from build123d import *

# Parameters (mm, degrees)
F0_R     = 1
F1_DEPTH = 1
F2_R     = 3
F3_W     = 1.5266574919
F3_H     = 4.5481626876
F4_DEPTH = 0.5
F5_R     = 0.5


with BuildPart() as f1:
    # F0 (on Top) → F1 (new body)
    with BuildSketch(Plane.XY):
        with BuildLine():
            ThreePointArc((-35.1311429143, -3.4115522057), (-32.1311429143, -6.4115522057), (-29.1311429143, -3.4115522057))
            Line((-29.1311429143, -3.4115522057), (-35.1311429143, -3.4115522057))
        make_face()
        with BuildLine():
            Line((-35.1311429143, -3.4115522057), (-29.1311429143, -3.4115522057))
            ThreePointArc((-29.1311429143, -3.4115522057), (-32.1311429143, -0.4115522057), (-35.1311429143, -3.4115522057))
        make_face()
        with Locations((-32.1311429143, -2.1592592821)):
            Circle(F0_R, mode=Mode.SUBTRACT)
        with BuildLine():
            Line((-25.6311429143, -3.4115522057), (-29.1311429143, -3.4115522057))
            ThreePointArc((-29.1311429143, -3.4115522057), (-32.1311429143, -6.4115522057), (-35.1311429143, -3.4115522057))
            Line((-35.1311429143, -3.4115522057), (-38.6311429143, -3.4115522057))
            Line((-38.6311429143, -3.4115522057), (-38.6311429143, -16.4115522057))
            Line((-38.6311429143, -16.4115522057), (-25.6311429143, -16.4115522057))
            Line((-25.6311429143, -16.4115522057), (-25.6311429143, -3.4115522057))
        make_face()
    extrude(amount=F1_DEPTH)

    # F2
    f2_edges = [f1.edges().sort_by_distance(p)[0] for p in [
        (-25.631143, -3.411552, 0.5),
        (-25.631143, -16.411552, 0.5),
        (-38.631143, -3.411552, 0.5),
        (-38.631143, -16.411552, 0.5),
    ]]
    fillet(f2_edges, radius=F2_R)

    # F3 (on face) → F4 (join)
    with BuildSketch(Plane.XY.offset(1)):
        with Locations((-35.2431219071, -7.959790295)):
            Rectangle(F3_W, F3_H)
        with Locations((-29.0191639215, -7.959790295)):
            Rectangle(F3_W, F3_H)
        with BuildLine():
            Line((-28.0351451192, -12.3141705765), (-32.1311429143, -12.3141705765))
            Line((-32.1311429143, -12.3141705765), (-32.1311429143, -14.8540753871))
            add(Edge.make_bspline(
                [(-28.0351451192, -12.3141705765), (-28.9659189681, -13.232003587), (-29.6096801758, -15.267544426), (-32.1311429143, -14.8540753871)],
                knots=[0, 0, 0, 0, 4.8195761623, 4.8195761623, 4.8195761623, 4.8195761623], degree=3))
        make_face()
        with BuildLine():
            Line((-32.1311429143, -12.3141705765), (-36.2271407093, -12.3141705765))
            add(Edge.make_bspline(
                [(-36.2271407093, -12.3141705765), (-35.2963668605, -13.232003587), (-34.6526056528, -15.267544426), (-32.1311429143, -14.8540753871)],
                knots=[0, 0, 0, 0, 4.8195761623, 4.8195761623, 4.8195761623, 4.8195761623], degree=3))
            Line((-32.1311429143, -14.8540753871), (-32.1311429143, -12.3141705765))
        make_face()
    extrude(amount=F4_DEPTH)

    # F5
    f5_edges = [f1.edges().sort_by_distance(p)[0] for p in [
        (-36.006451, -5.685709, 1.25),
        (-34.479793, -5.685709, 1.25),
        (-34.479793, -10.233872, 1.25),
        (-36.006451, -10.233872, 1.25),
        (-28.255835, -5.685709, 1.25),
        (-28.255835, -10.233872, 1.25),
        (-29.782493, -5.685709, 1.25),
        (-29.782493, -10.233872, 1.25),
        (-36.227141, -12.314171, 1.25),
        (-28.035145, -12.314171, 1.25),
    ]]
    fillet(f5_edges, radius=F5_R)


solid = f1.part
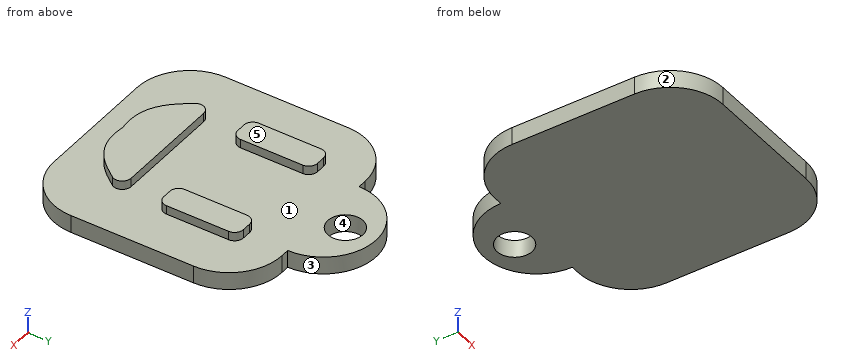
CAD build for the part. Positions are in the model's coordinates, mm. Face numbers are marked on the shaded views. A direction names the side the tool comes from. Coordinates: 2 decimals unless noted, no trailing zeros. Write each loop counter-clockwise with the first axis right and the second up, starting at its lowest first coordinate (ties: lowest second). Pieces come first, ordered by that corner, then holes. Notation, with made-up numbers: (63.5, 75) - (70.5, 75) arc R29 ccw to (70.5, 95) - close; hole circle Ø2 at (77.5, -26). An arc over 180 degrees is marked (long way). Use a Markdown table: item, result. Add a question column.
Item 1: Band-saw the part on B-B, the plane y = -11.5. Give the cut face in (x, z).
Item 2: Band-saw the part on C-C, the plane x = -37.5. Give the cut face in (y, z).
Item 3: 3-axis set-ups, long thin cutter, end or side, ignore diameter. For the marked faces 1 and 2: which of +Z, -Z, +X, -X, +Y, -Y reach the whole face in a straight line?
Item 4: Drill centre lines: L1, parallel to X at y = -6.25, z = 1.2; L2, parallel to Z at x = -31, y = -1.25; L3, parallel to Y at x = -35.25, z = 0.4. Where is each one in solid material? Low to high. Write a range as from..to.
Item 5: Mould opens along X. For the marked faces 3, 4 and 5 say: pulls with the +X half, pulls with the -X half, needs draft (parallel to the pull), parting line crosses it, or undercut.
Item 6: Flat gauge pins, fed straight in: pin 1 (5 mm diameter, centred on x = -37, y = -5.5, fed in from -Z); pin 2 (0.6 mm diameter, centred on x = -35, z = 1.5, fed in from -Y); pin 3 (2.5 mm diameter, centred on x = -32.13, y = -2.16, fed in from +Z); pin 4 (0.6 mm diameter, centred on x = -29, z = 1.5, fed in from +Y). Where does each tip first touch, or does it go through?
Item 7: Band-saw the part on A-A, the plane z = 0.7. Give the cut face in (x, y), and give its area (3 significant figures).
Numbers:
| question | item | result |
|---|---|---|
| 1 | outline | (-38.63, 0) - (-25.63, 0) - (-25.63, 1) - (-38.63, 1) - close |
| 2 | outline | (-15.76, 0) - (-4.06, 0) - (-4.06, 1) - (-15.76, 1) - close |
| 3 | face 1 | +Z |
| 3 | face 2 | +Z, -Z, -X, -Y |
| 4 | L1 | -36.01..-34.48, -29.78..-28.26 |
| 4 | L2 | 0..1 |
| 4 | L3 | -16.41..-3.41 |
| 5 | face 3 | parting line crosses it |
| 5 | face 4 | undercut |
| 5 | face 5 | needs draft |
| 6 | pin 1 | z = 0 |
| 6 | pin 2 | y = -14.15 |
| 6 | pin 3 | z = 1 |
| 6 | pin 4 | y = -5.69 |
| 7 | outline | (-38.63, -13.41) arc R3 ccw to (-35.63, -16.41) - (-28.63, -16.41) arc R3 ccw to (-25.63, -13.41) - (-25.63, -6.41) arc R3 ccw to (-28.63, -3.41) - (-29.13, -3.41) arc R3 ccw to (-35.13, -3.41) - (-35.63, -3.41) arc R3 ccw to (-38.63, -6.41) - close; hole circle Ø2 at (-32.13, -2.16) |
| 7 | area | 172 mm2 |
